Verification items for this drawing (mm, ordinates from the low corner). Give positions to 0.01 mm unless a question says otherwise; leave off trailing zeros. Loops run counter-clockwise (first coordinate to the right, second up) from the corner with the lowest first, then second, coordinate; pieces in that order, holes last. Notation, with made-up numbers: (44.25, -33.5) -> (65.25, -33.5) arc R23 ccw to (65.25, 0.5) -> close; hole circle Ø10 at (23, 56). An arc over 180 degrees is marked (long way). Answer in a Markdown table with one row per item. Add a question column.
Q1. Section check B-B on z = 48.5. Enter the section's corners in (x, y), and give its area (3 significant figures).
Q2. Section check C-C on x = 37.5. Enter the section's corners in (y, z).
Q3. Gauge pin test, flat ends, axial feed: P1, Ø8, axis at y = 5.5, z = 33.5, coming from the -X side; P2, Ø10.5, axis at x = 42.5, z = 53.5, coming from the +Y side; P3, Ø5, axis at x = 11.5, z = 67, coming from the +Y side. Record the tip position at first contact, or that the pin passes through.
Q4. Release check for a two-part mould opening along X. For the marked faces 1 and 2 record: pulls with the +X half, pulls with the -X half, needs draft (parallel to the pull), parting line crosses it, or undercut.
Q5. Section check D-D on y = 22. Enter the section's corners in (x, z).
Q6. Material ranges on probe 1 along Z at (x, y) = (48, 4); probe 2 along X at (y, z) = (6, 50); probe 3 along X at (y, z) = (11, 46.5), recorded low to high.
Q7. Section check A-A on x = 48.5. Enter the section's corners in (y, z).
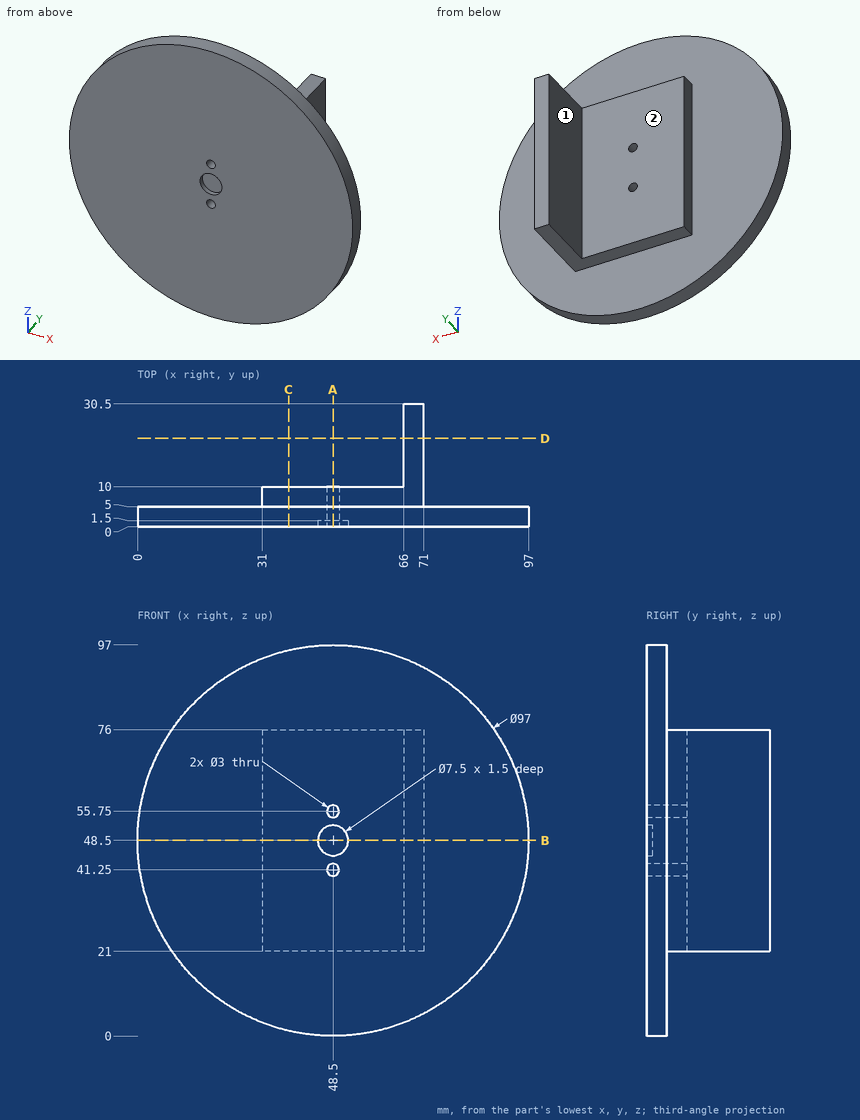
Taken from the geometry:
| question | item | result |
|---|---|---|
| 1 | outline | (0, 0) -> (44.75, 0) -> (44.75, 1.5) -> (52.25, 1.5) -> (52.25, 0) -> (97, 0) -> (97, 5) -> (71, 5) -> (71, 30.5) -> (66, 30.5) -> (66, 10) -> (31, 10) -> (31, 5) -> (0, 5) -> close |
| 1 | area | 776 mm² |
| 2 | outline | (0, 1.26) -> (5, 1.26) -> (5, 21) -> (10, 21) -> (10, 76) -> (5, 76) -> (5, 95.74) -> (0, 95.74) -> close |
| 3 | P1 | stops at x = 1.27 |
| 3 | P2 | stops at y = 10 |
| 3 | P3 | stops at y = 5 |
| 4 | face 1 | pulls with the -X half |
| 4 | face 2 | needs draft |
| 5 | outline | (66, 21) -> (71, 21) -> (71, 76) -> (66, 76) -> close |
| 6 | probe 1 | z = 0 to 39.84, 42.66 to 54.34, 57.16 to 97 |
| 6 | probe 2 | x = 31 to 71 |
| 6 | probe 3 | x = 66 to 71 |
| 7 | outline | (0, 0) -> (5, 0) -> (5, 21) -> (10, 21) -> (10, 39.75) -> (0, 39.75) -> close; (0, 42.75) -> (10, 42.75) -> (10, 54.25) -> (0, 54.25) -> (0, 52.25) -> (1.5, 52.25) -> (1.5, 44.75) -> (0, 44.75) -> close; (0, 57.25) -> (10, 57.25) -> (10, 76) -> (5, 76) -> (5, 97) -> (0, 97) -> close |
